The figure shows three views and two pictorial views of one solid part (mm, origin at its lowest corner). Answer the questions. A direction names the side the tool comes from. Round coordinates to 2 decimals unless told otherwise and drop trailing zeros. Write each loop counter-clockwise with the first axis right and the second up, starting at its lowest first coordinate (ties: lowest second). Pieces come first, ordered by that corner, then holes. Notation, with made-up numbers: M 82,8.5 L 118,8.5 A19 cw 118,27.5 Z; hole C 14.25,-30.5 d10. An arc over 180 degrees is marked long. Use one line per item in the form item = value. Start each with the question number.
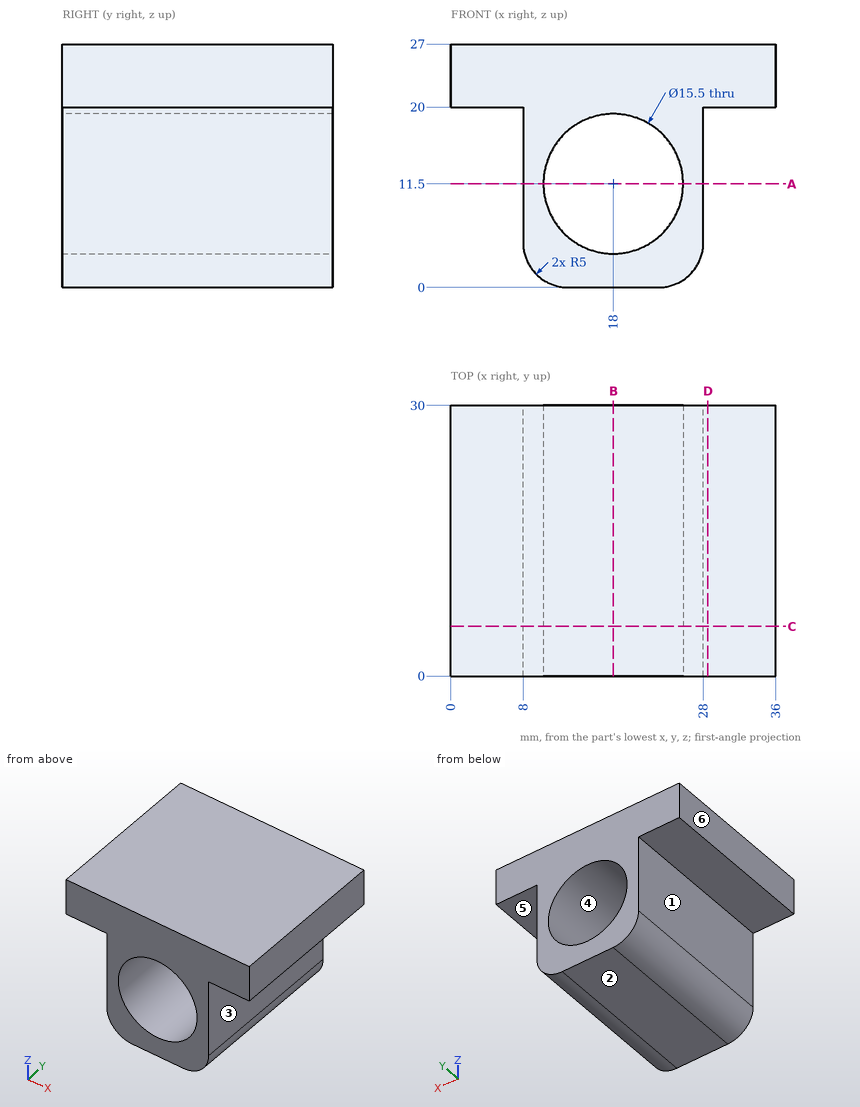
Q1. Find section A-A on z = 11.5. Write down the section's boundary in (x, y), and give its area (3 significant figures).
Q2. Straight lines are drawn through the part: line 1 (X direction, y = 24.25, z = 11.5); line 2 (X direction, y = 17, z = 7); line 3 (Z direction, x = 23, y = 21.25). For each, find the intervals that lie inside material, in ascending order. Write a range as [from, to].
Q3. Find section D-D on x = 28.5. Write down the section's boundary in (y, z), and give its area (3 significant figures).
Q4. A tool of negligible diameter and unlimited length cuts with its end or side. For the marked faces 1 and 2, from which of +Z, -Z, +X, -X, +Y, -Y can it reach the whole face along a straight path? Write none if from no direction.
Q5. Find section B-B on x = 18. Write down the section's boundary in (y, z), and give its area (3 significant figures).
Q6. For a pull along X with two mould halves and no side action, classify the marked faces 3, 4, 5 and 6 as +X half, -X half, draft (parallel to the pull), parting line (faces both ways), or undercut.
Q7. Find section C-C on y = 5.5. Write down the section's boundary in (x, z).
Q8. Each of these flat-tipped pins is pushed along its axis until it touches: pin 1 Ø1.5 at (x, z) = (28, 22.5) entering from -Y; pin 2 Ø12.5 at (x, z) = (18, 11.5) entering from -Y; pin 3 Ø4 at (x, y) = (2, 9) entering from -Z; pin 4 Ø1 at (y, z) = (10, 12) entering from -X. Where does it stop, or does it pass through?
Response:
q1.outline = M 8,0 L 10.25,0 L 10.25,30 L 8,30 Z; M 25.75,0 L 28,0 L 28,30 L 25.75,30 Z
q1.area = 135 mm²
q2.line_1 = [8, 10.25], [25.75, 28]
q2.line_2 = [8, 11.69], [24.31, 28]
q2.line_3 = [0, 5.58], [17.42, 27]
q3.outline = M 0,20 L 30,20 L 30,27 L 0,27 Z
q3.area = 210 mm²
q4.face_1 = -Z, -X, +Y, -Y
q4.face_2 = -Z, +X, -X, +Y, -Y
q5.outline = M 0,0 L 30,0 L 30,3.75 L 0,3.75 Z; M 0,19.25 L 30,19.25 L 30,27 L 0,27 Z
q5.area = 345 mm²
q6.face_3 = +X half
q6.face_4 = undercut
q6.face_5 = draft
q6.face_6 = -X half
q7.outline = M 0,20 L 8,20 L 8,5 A5 ccw 13,0 L 23,0 A5 ccw 28,5 L 28,20 L 36,20 L 36,27 L 0,27 Z; hole C 18,11.5 d15.5
q8.pin_1 = 0
q8.pin_2 = through
q8.pin_3 = 20
q8.pin_4 = 8
